Autodesk Inventor part; units mm, degrees
ref_plane "YZ Plane" through (0, 0, 0) normal (1, 0, 0) x (0, 1, 0)
ref_plane "XZ Plane" through (0, 0, 0) normal (0, 1, 0) x (-1, 0, 0)
ref_plane "XY Plane" through (0, 0, 0) normal (0, 0, 1) x (1, 0, 0)
sketch "Esboço1" plane through (0, 0, 0) normal (0, 1, 0) x (-1, 0, 0)
  line L0 (0, 0) -> (40, 0)
  line L1 (40, 0) -> (40, -20)
  line L2 (40, -20) -> (0, -20)
  line L3 (0, -20) -> (0, 0)
  dimension "d0" = 40
  dimension "d1" = 20
extrude "Extrusão1" add sketch "Esboço1" along normal blind 3
sketch "Esboço2" plane through (0, 3, 0) normal (0, 1, 0) x (1, 0, 0)
  circle A0 centre (-30, 10.0153) radius 1.5
  circle A1 centre (-10, 10.0153) radius 1.5
  line L0 (-40, 20) -> (-40, 0)
  line L1 (0, 0) -> (0, 20)
  dimension "d5" = 3
  dimension "d6" = 3
  dimension "d7" = 10
  dimension "d8" = 10
extrude "Extrusão2" add sketch "Esboço2" along normal blind 28.5
Could you check a few things on this model? Use its own coordinates, in mm. A direction names the side the tool comes from. Coordinates: 2 decimals unless noted, no trailing zeros. Order: outer loops, then holes, each group sorted by start corner. A loop starts at its lowest first (then second) coordinate and runs counter-clockwise, first axis right, second up. Notation, with made-up numbers: M 85,44 L 116,44 A25 ccw 116,70 Z; hole C -14,-15.75 d9. An arc over 180 degrees is marked long. Use one line per item in the form item = value. Start each with the question number.
1. Suppose I cut it at B-B on z = -10.5. Write out the boundary of the cut face in (x, y).
2. For pin 1 (10 mm diameter, centred on y = 27, z = -5.5, fed in from +X); pin 2 (2 mm diameter, centred on x = -6, z = -11, fed in from +Y); pin 3 (3 mm diameter, centred on x = -9.5, y = 5.5, fed in from -Z), each with a flat end and sliding along its axis, tell me the tip position at first contact or that it passes through.
3. On a 3-axis mill with a long thin cutter (end or side, diameter ignored), from which of +Z, -Z, +X, -X, +Y, -Y can I reach the whole of each face in a straight line? I mean faces 1 (the cylindrical face through (-11.106, 17.05, -9.002)), 2 (the flat face through (-30, 31.5, -10)). Say none if no direction works.
4. Suppose I cut it at A-A on x = -30. Write out the boundary of the cut face in (y, z), then the cut area to 4 significant figures.
5. We'd pull the mould along X, two halves only. Please class faces 3 (the flat face through (0, 1, -10)), 4 (the flat face through (-10, 31.5, -10)), 5 (the cylindrical face through (-31.5, 17.05, -9.95)): +X half, -X half, draft (parallel to the pull), parting line (faces both ways), or undercut.
6. Suppose I cut it at D-D on x = -12.5. Write out the boundary of the cut face in (y, z), then the cut area to 3 significant figures.
7. Please list where these lines run through material, in increasing order: line 1 (Y direction, x = -25, z = -18.25); line 2 (Z direction, x = -11, y = 25).
8. Suppose I cut it at C-C on y = 28. Write out the boundary of the cut face in (x, z), then the cut area to 3 significant figures.
Geometry says:
q1.outline = M -40,0 L 0,0 L 0,3 L -8.58,3 L -8.58,31.5 L -11.42,31.5 L -11.42,3 L -28.58,3 L -28.58,31.5 L -31.42,31.5 L -31.42,3 L -40,3 Z
q2.pin_1 = -8.5
q2.pin_2 = 3
q2.pin_3 = -11.52
q3.face_1 = +Y
q3.face_2 = +Z, -Z, +X, -X, +Y
q4.outline = M 0,-20 L 3,-20 L 3,-11.52 L 31.5,-11.52 L 31.5,-8.52 L 3,-8.52 L 3,0 L 0,0 Z
q4.area = 145.5 mm^2
q5.face_3 = +X half
q5.face_4 = draft
q5.face_5 = undercut
q6.outline = M 0,-20 L 3,-20 L 3,0 L 0,0 Z
q6.area = 60.0 mm^2
q7.line_1 = 0 to 3
q7.line_2 = -11.13 to -8.9
q8.outline = C -30,-10.02 d3; C -10,-10.02 d3
q8.area = 14.1 mm^2
